Geometry: final body of the model. Coordinates: model frame, mm. Face numbers are marked on the shaded views. A direction names the side the tool comes from. Give positions to 0.01 mm unless a question says otherwise; leave off trailing zeros. Loops run counter-clockwise (first coordinate to the right, second up) from the corner with the lowest first, then second, coordinate; pieces in that order, holes last.
1. Section C-C, the plane z = 14.75. Output: boundary loops of the cut face in (x, y).
2. First-contact query: P1, Ø1.3, axis at x = 0.5, z = -3.5, coming from the -Y side; P2, Ø3, axis at x = 0, y = 0, coming from the +Z side; P3, Ø0.8, axis at y = 0.5, z = -2.5, coming from the +X side. Flat tips, straight axial feed; report the tip coordinate or a pass-through.
3. Draft query along X for the marked faces 1, 2, 3 and 4. Return one class per face: +X half, -X half, draft (parallel to the pull), parting line (faces both ways), or undercut.
4. Section B-B, the plane z = 4.5. Output: boundary loops of the cut face in (x, y).
5. Section A-A, the plane z = -2.75. Output: boundary loops of the cut face in (x, y).
6. Material intervals for line 1 along Y through (x, z) = (0, 10); line 2 along Z through (x, y) = (2, 0.75); line 3 along Y through (x, z) = (-1, 10.75), sorted ascending.
7. Access query for the marked faces 5, 6 and 7. Directions: +Z, -Z, +X, -X, +Y, -Y. A direction counts if a zero-diameter tool reaches every point of the face in a straight line with its end or side. Return the directions, or none.
8. Section D-D, the plane y = -6.75. Output: boundary loops of the cut face in (x, z).
from build123d import *

# Parameters (mm, degrees)
SKETCH1_R           = 5
BOSS_EXTRUDE1_DEPTH = 9.8
SKETCH2_R           = 7.85
BOSS_EXTRUDE2_DEPTH = 1.5
SKETCH3_R           = 5
BOSS_EXTRUDE3_DEPTH = 9.4
SKETCH4_W           = 2.5
SKETCH4_H           = 0.8
SKETCH4_W_2         = 0.8
SKETCH4_H_2         = 2.5
BOSS_EXTRUDE4_DEPTH = 7.1
FILLET1_R           = 1
SKETCH6_R           = 2.8
CUT_EXTRUDE1_DEPTH  = 15
SKETCH7_R           = 1.25
BOSS_EXTRUDE5_DEPTH = 8
CHAMFER1_SIZE       = 1
CHAMFER2_SIZE       = 0.5


with BuildPart() as part:
    # Sketch1 → Boss-Extrude1 (new body)
    with BuildSketch(Plane.XY):
        Circle(SKETCH1_R)
    extrude(amount=BOSS_EXTRUDE1_DEPTH)

    # Sketch2 → Boss-Extrude2 (add)
    with BuildSketch(Plane.XY.offset(9.8)):
        Circle(SKETCH2_R)
    extrude(amount=-BOSS_EXTRUDE2_DEPTH)

    # Sketch3 → Boss-Extrude3 (add)
    with BuildSketch(Plane.XY.offset(9.8)):
        Circle(SKETCH3_R)
    extrude(amount=BOSS_EXTRUDE3_DEPTH)

    # Sketch4 → Boss-Extrude4 (add)
    with BuildSketch(Plane(origin=(0, 0, 0), x_dir=(-1, 0, 0), z_dir=(0, 0, -1))):
        with Locations((0, 2.9)):
            Rectangle(SKETCH4_W, SKETCH4_H)
        with Locations((3.285473872, 0)):
            Rectangle(SKETCH4_W_2, SKETCH4_H_2)
        Polygon((-3.130059347, -1.992660833), (-3.391380505, 0.493643905), (-2.595762989, 0.577266676), (-2.33444183, -1.909038062), align=None)
    extrude(amount=BOSS_EXTRUDE4_DEPTH)

    # Fillet1
    fillet1_edges = [part.edges().sort_by_distance(p)[0] for p in [
        (1.25, 2.9, -7.1),
        (-1.25, 2.9, -7.1),
        (-3.285473872, 1.25, -7.1),
        (-3.285473872, -1.25, -7.1),
        (2.732250589, -1.950849448, -7.1),
        (2.993571747, 0.535455291, -7.1),
    ]]
    fillet(fillet1_edges, radius=FILLET1_R)

    # Sketch6 → Cut-Extrude1 (cut)
    with BuildSketch(Plane.XY.offset(19.2)):
        Circle(SKETCH6_R)
    extrude(amount=-CUT_EXTRUDE1_DEPTH, mode=Mode.SUBTRACT)

    # Sketch7 → Boss-Extrude5 (add)
    with BuildSketch(Plane.XY.offset(4.2)):
        Circle(SKETCH7_R)
    extrude(amount=BOSS_EXTRUDE5_DEPTH)

    # Chamfer1
    chamfer1_edges = [part.edges().sort_by_distance(p)[0] for p in [
        (-5, 0, 19.2),
    ]]
    chamfer(chamfer1_edges, length=CHAMFER1_SIZE)

    # Chamfer2
    chamfer2_edges = [part.edges().sort_by_distance(p)[0] for p in [
        (-2.8, 0, 19.2),
    ]]
    chamfer(chamfer2_edges, length=CHAMFER2_SIZE)


solid = part.part
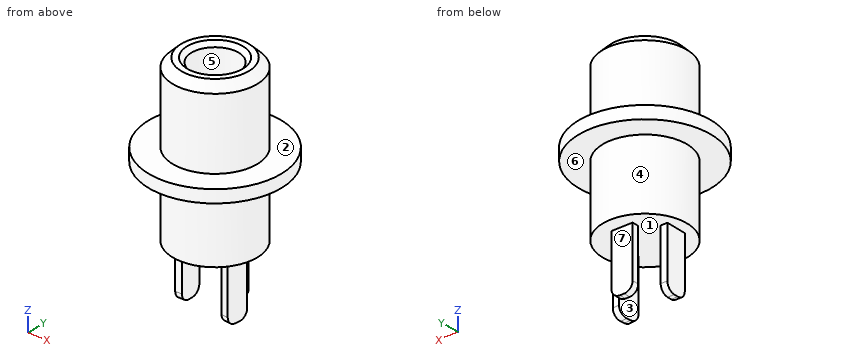
Answers below:
1. outline: circle Ø10 at (0, 0); hole circle Ø5.6 at (0, 0)
2. P1: stops at y = 2.5
2. P2: stops at z = 12.2
2. P3: stops at x = 3.39
3. face 1: undercut
3. face 2: draft
3. face 3: undercut
3. face 4: parting line
4. outline: circle Ø10 at (0, 0); circle Ø2.5 at (0, 0); hole circle Ø5.6 at (0, 0)
5. outline: (-3.69, -1.25) - (-2.89, -1.25) - (-2.89, 1.25) - (-3.69, 1.25) - close; (-1.25, 2.5) - (1.25, 2.5) - (1.25, 3.3) - (-1.25, 3.3) - close; (2.33, -1.91) - (3.13, -1.99) - (3.39, 0.49) - (2.6, 0.58) - close
6. line 1: y = -5 to -2.8, -1.25 to 1.25, 2.8 to 5
6. line 2: z = 0 to 4.2
6. line 3: y = -4.9 to -2.62, -0.75 to 0.75, 2.62 to 4.9
7. face 5: +Z
7. face 6: -Z
7. face 7: -Z, +X, -X, +Y
8. outline: (-4.01, 8.3) - (4.01, 8.3) - (4.01, 9.8) - (-4.01, 9.8) - close
